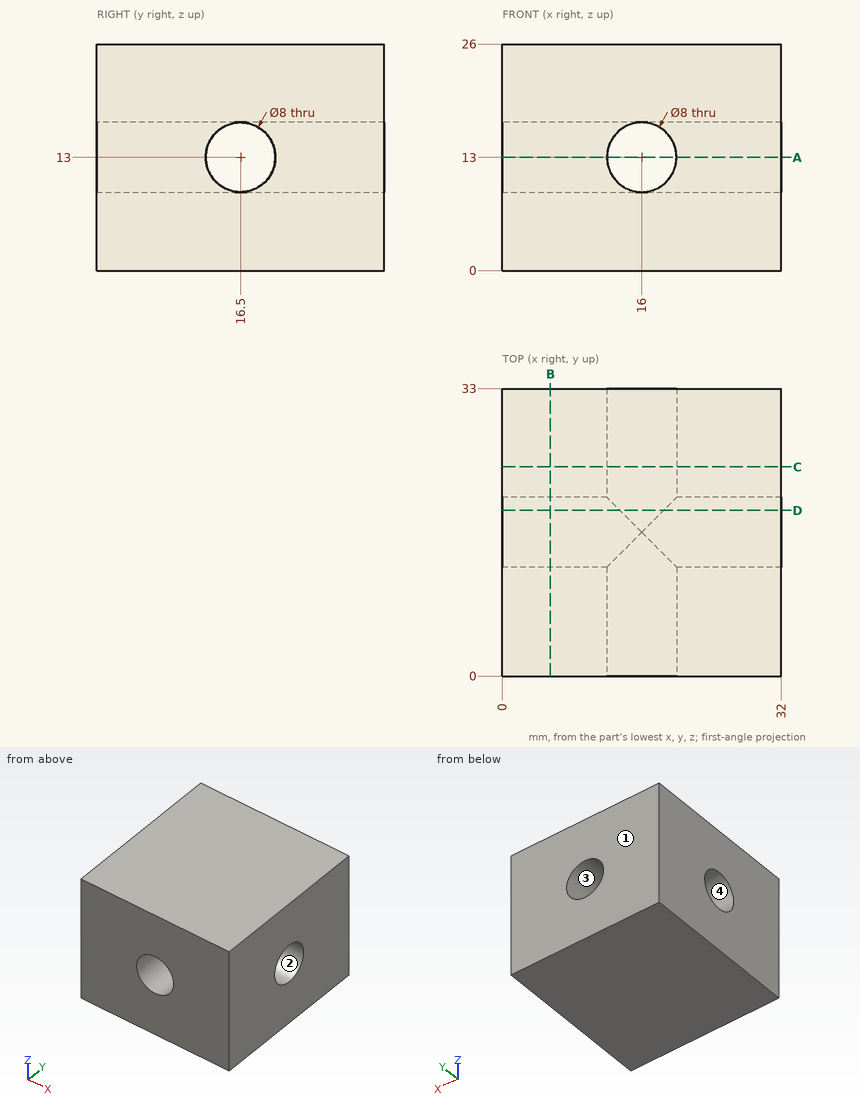
Input: dimensioned drawing with shaded views. Units: mm. Origin: part minimum x, y, z. Coordinates: 2 decimals unless noted, no trailing zeros. Order: outer loops, then holes, each group sorted by start corner. A loop starts at its lowest first (then second) coordinate and runs counter-clockwise, first axis right, second up.
1. Draft query along Y for the marked faces 1, 2, 3 and 4. Return one class per face: +Y half, -Y half, draft (parallel to the pull), parting line (faces both ways), or undercut.
Checked values:
face 1: +Y half
face 2: undercut
face 3: draft
face 4: undercut
2. Contact query for a flat-ended pin moving along its axis: P1, Ø13, axis at x = 16, z = 13, coming from the -Y side. Output: stop coordinate, or through.
Checked values:
P1: stops at y = 0
3. Cut plane A-A, the plane z = 13. Return loops of the section in (x, y), plus the area to 3 significant figures.
Checked values:
outline: (0, 0) - (12, 0) - (12, 12.5) - (0, 12.5) - close; (0, 20.5) - (12, 20.5) - (12, 33) - (0, 33) - close; (20, 0) - (32, 0) - (32, 12.5) - (20, 12.5) - close; (20, 20.5) - (32, 20.5) - (32, 33) - (20, 33) - close
area: 600 mm2
4. Cut plane B-B, the plane x = 5.5. Return loops of the section in (y, z).
Checked values:
outline: (0, 0) - (33, 0) - (33, 26) - (0, 26) - close; hole circle Ø8 at (16.5, 13)
5. Ray query, line 1 along Z through (x, y) = (16, 13); line 2 along Y through (x, z) = (3.5, 12.75); line 3 along X through (y, z) = (9, 13). Return the intervals inside material, ascending.
Checked values:
line 1: z = 0 to 9, 17 to 26
line 2: y = 0 to 12.51, 20.49 to 33
line 3: x = 0 to 12, 20 to 32
6. Cut plane C-C, the plane y = 24. Return loops of the section in (x, z).
Checked values:
outline: (0, 0) - (32, 0) - (32, 26) - (0, 26) - close; hole circle Ø8 at (16, 13)
7. Cut plane D-D, the plane y = 19. Return loops of the section in (x, z).
Checked values:
outline: (0, 0) - (32, 0) - (32, 9.88) - (18.5, 9.88) arc R4 cw to (13.5, 9.88) - (0, 9.88) - close; (0, 16.12) - (13.5, 16.12) arc R4 cw to (18.5, 16.12) - (32, 16.12) - (32, 26) - (0, 26) - close
